Geometry: final body of the model. Coordinates: model frame, mm. A direction names the side the tool comes from. Coordinates: 2 decimals unless noted, no trailing zeros. Loops run counter-clockwise (first coordinate to the right, second up) from the corner with the lowest first, then second, coordinate; pieces in that order, holes last. Notation, with made-up numbers: (-28, -12.75) - (-3, -12.75) arc R12 ccw to (-3, -2.75) - close; hole circle Ø9 at (54.25, 16.25). An arc over 180 degrees is marked (long way). Answer in a Markdown table with one row per item.
from build123d import *

# Parameters (mm, degrees)
F0_W     = 145.3911811113
F0_H     = 100.7209792733
F2_DEPTH = 63.5
F1_R     = 21.0519907021
F1_R_2   = 10.1625017611
F3_DEPTH = 80.01
F4_DEPTH = 127
F5_R     = 5.08


with BuildPart() as f2:
    # F0 (on Front) → F2 (new body, symmetric)
    with BuildSketch(Plane.XZ):
        Rectangle(F0_W, F0_H)
    extrude(amount=F2_DEPTH, both=True)

    # F1 (on face) → F3 (join)
    with BuildSketch(Plane.XZ):
        Circle(F1_R)
        Circle(F1_R_2, mode=Mode.SUBTRACT)
    extrude(amount=F3_DEPTH)

    # F4 (cut): a face of the model
    f4_faces = [f2.faces().sort_by_distance(p)[0] for p in [
        (0, -63.5, 0),
    ]]
    extrude(f4_faces, amount=-F4_DEPTH, mode=Mode.SUBTRACT)

    # F5
    f5_edges = [f2.edges().sort_by_distance(p)[0] for p in [
        (0, -63.5, 50.36049),
        (-72.695591, -63.5, 0),
        (0, -63.5, -50.36049),
        (72.695591, -63.5, 0),
        (-21.051991, -63.5, 0),
        (0, 63.5, 50.36049),
        (-72.695591, 0, 50.36049),
        (72.695591, 0, 50.36049),
        (-72.695591, 63.5, 0),
        (-72.695591, 0, -50.36049),
        (72.695591, 63.5, 0),
        (72.695591, 0, -50.36049),
        (-21.051991, -80.01, 0),
        (0, 63.5, -50.36049),
        (-10.162502, 63.5, 0),
    ]]
    fillet(f5_edges, radius=F5_R)


solid = f2.part
(1) Access query for faces 1 (the face through (-16, 63.5, 1)), 2 (the face through (-4.564, -71.711, -20.551)). Directions: +Z, -Z, +X, -X, +Y, -Y. A direction counts if a zero-diameter tool reaches every point of the face in a straight line with its end or side. Return the directions, or none.
Verdict:
| item | result |
|---|---|
| face 1 | +Z, -Z, +X, -X, +Y |
| face 2 | -Y |
(2) First-contact query: pin 1 Ø2 at (x, z) = (-25.5, -30) entering from -Y; pin 2 Ø1 at (x, z) = (-17.5, -14) entering from -Y. Flat tips, straight axial feed; report the tip coordinate or a pass-through.
Verdict:
| item | result |
|---|---|
| pin 1 | stops at y = -63.5 |
| pin 2 | stops at y = -65.75 |
(3) Cut plane A-A on x = 0. Output: boundary loops of the cut face in (y, z).
Verdict:
| item | result |
|---|---|
| outline | (-80.01, -15.97) arc R5.08 ccw to (-74.93, -21.05) - (-68.58, -21.05) arc R5.08 cw to (-63.5, -26.13) - (-63.5, -45.28) arc R5.08 ccw to (-58.42, -50.36) - (58.42, -50.36) arc R5.08 ccw to (63.5, -45.28) - (63.5, -15.24) arc R5.08 ccw to (58.42, -10.16) - (-80.01, -10.16) - close; (-80.01, 10.16) - (58.42, 10.16) arc R5.08 ccw to (63.5, 15.24) - (63.5, 45.28) arc R5.08 ccw to (58.42, 50.36) - (-58.42, 50.36) arc R5.08 ccw to (-63.5, 45.28) - (-63.5, 26.13) arc R5.08 cw to (-68.58, 21.05) - (-74.93, 21.05) arc R5.08 ccw to (-80.01, 15.97) - close |
(4) Cut plane C-C on y = -45. Output: boundary loops of the cut face in (x, z) (1 decimal).
Verdict:
| item | result |
|---|---|
| outline | (-72.7, -45.3) arc R5.1 ccw to (-67.6, -50.4) - (67.6, -50.4) arc R5.1 ccw to (72.7, -45.3) - (72.7, 45.3) arc R5.1 ccw to (67.6, 50.4) - (-67.6, 50.4) arc R5.1 ccw to (-72.7, 45.3) - close; hole circle Ø20.3 at (0, 0) |
(5) Ray query, probe 1 along Z at (x, y) = (0, 5.5); probe 2 along X at (y, z) = (13, 0); probe 3 along Y at (x, z) = (47.5, 12). Return the intervals inside material, ascending.
Verdict:
| item | result |
|---|---|
| probe 1 | z = -50.36 to -10.16, 10.16 to 50.36 |
| probe 2 | x = -72.7 to -10.16, 10.16 to 72.7 |
| probe 3 | y = -63.5 to 63.5 |
(6) Cut plane D-D on x = -40.5. Output: boundary loops of the cut face in (y, z), then the cut area to 3 significant figures.
Verdict:
| item | result |
|---|---|
| outline | (-63.5, -45.28) arc R5.08 ccw to (-58.42, -50.36) - (58.42, -50.36) arc R5.08 ccw to (63.5, -45.28) - (63.5, 45.28) arc R5.08 ccw to (58.42, 50.36) - (-58.42, 50.36) arc R5.08 ccw to (-63.5, 45.28) - close |
| area | 12,800 mm² |
(7) Cut plane B-B on z = 0. Output: boundary loops of the cut face in (x, y).
Verdict:
| item | result |
|---|---|
| outline | (-72.7, -58.42) arc R5.08 ccw to (-67.62, -63.5) - (-26.13, -63.5) arc R5.08 cw to (-21.05, -68.58) - (-21.05, -74.93) arc R5.08 ccw to (-15.97, -80.01) - (-10.16, -80.01) - (-10.16, 58.42) arc R5.08 ccw to (-15.24, 63.5) - (-67.62, 63.5) arc R5.08 ccw to (-72.7, 58.42) - close; (10.16, -80.01) - (15.97, -80.01) arc R5.08 ccw to (21.05, -74.93) - (21.05, -68.58) arc R5.08 cw to (26.13, -63.5) - (67.62, -63.5) arc R5.08 ccw to (72.7, -58.42) - (72.7, 58.42) arc R5.08 ccw to (67.62, 63.5) - (15.24, 63.5) arc R5.08 ccw to (10.16, 58.42) - close |
